Read the model definition and answer for the solid it produces. Units are mm, in the model's axes. A direction names the side the tool comes from. Give positions to 0.01 mm unless a question says otherwise; leave off trailing zeros. Order: outer loops, then holes, each group sorted by start corner. A loop starts at its lowest first (then second) coordinate and runs counter-clockwise, first axis right, second up. Notation, with made-up numbers: (50, 37.5) - (76, 37.5) arc R29 ccw to (76, 65.5) - close; hole circle Ø3 at (-17, 55.5). An arc over 180 degrees is marked (long way). Answer as CSV lines item,"result". Start each with the question number.
from build123d import *

# Parameters (mm, degrees)
F0_R     = 1.5
F1_DEPTH = 3
F3_DEPTH = 6
F4_R     = 1.5
F5_DEPTH = 25
F7_DEPTH = 25


with BuildPart() as f1:
    # F0 (on Front) → F1 (new body)
    with BuildSketch(Plane.XZ):
        Polygon((16.378661, 45), (0, 0), (40, 0), (46.378661, 45), align=None)
        with Locations((19.878661, 41.5)):
            Circle(F0_R, mode=Mode.SUBTRACT)
        with BuildLine():
            ThreePointArc((43.378661, 41.5), (42.577917, 35.417752), (40.230258, 29.75))
            ThreePointArc((40.230258, 29.75), (38.181219, 29.200962), (37.632181, 31.25))
            ThreePointArc((37.632181, 31.25), (39.68014, 36.19421), (40.378661, 41.5))
            ThreePointArc((40.378661, 41.5), (41.878661, 43), (43.378661, 41.5))
        make_face(mode=Mode.SUBTRACT)
    extrude(amount=F1_DEPTH)

    # F2 (on face) → F3 (join)
    with BuildSketch(Plane(origin=(0, 0, 0), x_dir=(-1, 0, 0), z_dir=(0, 1, 0))):
        Polygon((-40.425244, 3), (-40, 0), (-2, 0), (-2, 3), align=None)
    extrude(amount=F3_DEPTH)

    # F4 (on face) → F5 (cut)
    with BuildSketch(Plane(origin=(0, 0, 0), x_dir=(1, 0, 0), z_dir=(0, 0, -1))):
        with Locations((37, -3)):
            Circle(F4_R)
        with Locations((5, -3)):
            Circle(F4_R)
    extrude(amount=-F5_DEPTH, mode=Mode.SUBTRACT)

    # F6 (on face) → F7 (cut)
    with BuildSketch(Plane.XZ.offset(3)):
        Polygon((18.830264, 34.192898), (8.568888, 6), (26.311674, 6), align=None)
        Polygon((40, 21), (22.968705, 34.192898), (30.450115, 6), (35.450115, 6), align=None)
        with BuildLine():
            ThreePointArc((24.878661, 41.5), (24.70829, 40.205905), (24.208788, 39))
            Line((24.208788, 39), (34.601092, 33))
            ThreePointArc((34.601092, 33), (36.2994, 37.100076), (36.878661, 41.5))
            Line((36.878661, 41.5), (24.878661, 41.5))
        make_face()
    extrude(amount=-F7_DEPTH, mode=Mode.SUBTRACT)


with BuildPart() as f8_1:
    # F8: instance of F1
    add(f1.part.mirror(Plane(origin=(24.806781, -3, 21.611158), x_dir=(1, 0, 0), z_dir=(0, -1, 0))))


solid = f8_1.part
(1) Determine the mould class of faces 4 (the flat face through (20, -7, 0)), 5 (the flat face through (8.3, -4.5, 22.8)), 6 (the cylindrical face through (41.85, -4.52, 43)), 7 (the flat face through (21, -12, 2)) for opening direction Z: released by +Z, released by -Z, zero draft, split by the parting line, or undercut.
(2) Section C-C, the plane x = 15 is taken. Write down the section's boundary in (y, z), and give its area (3 significant figures).
(3) Flat-ended cylindrical pins translate along their axes: pin 1 Ø2.5 at (x, y) = (29, -4) entering from -Z; pin 2 Ø2.5 at (x, y) = (5, -9) entering from -Z; pin 3 Ø1.5 at (y, z) = (-4, 15.5) entering from -X; pin 4 Ø8 at (x, z) = (14.5, 17) entering from -Y. Find the tip coordinate at first contact, or state that the pin passes through.
(4) Section D-D, the plane z = 16 is taken. Write down the section's boundary in (x, y).
(5) Straight lines are drawn through the part: line 1 (Y direction, x = 5, z = 1); line 2 (Z direction, x = 33.5, y = -5.25); line 3 (Y direction, x = 16.5, z = 34). For each, find the intervals that lie inside material, in ascending order. Write a range as [from, to].
(6) Section B-B, the plane z = 32 is taken. Write down the section's boundary in (x, y).
(7) Which of the six approach directions +Z, -Z, +X, -X, +Y, -Y give full straight-line access (tool end or side, diameter ignored) to faces 1 (the flat face through (23, -3, 23)), 2 (the cylindrical face through (39.66, -4.52, 36.12)), 3 (the flat face through (21, -9, 3))?
(8) Section A-A, the plane y = -9 is taken. Write down the section's boundary in (x, z).
Checks:
1,face 4,"released by -Z"
1,face 5,"released by +Z"
1,face 6,"undercut"
1,face 7,"zero draft"
2,outline,"(-12, 0) - (-3, 0) - (-3, 6) - (-6, 6) - (-6, 3) - (-12, 3) - close; (-6, 23.67) - (-3, 23.67) - (-3, 41.21) - (-6, 41.21) - close"
2,area,"88.6 mm²"
3,pin 1,"stops at z = 0"
3,pin 2,"passes through"
3,pin 3,"stops at x = 5.37"
3,pin 4,"stops at y = -6"
4,outline,"(5.82, -6) - (12.21, -6) - (12.21, -3) - (5.82, -3) - close; (23.66, -6) - (27.8, -6) - (27.8, -3) - (23.66, -3) - close; (38.48, -6) - (42.27, -6) - (42.27, -3) - (38.48, -3) - close"
5,line 1,"y = [-12, -10.5], [-7.5, -3]"
5,line 2,"z = [0, 6], [26.04, 33.64], [41.5, 45]"
5,line 3,"y = [-6, -3]"
6,outline,"(11.65, -6) - (18.03, -6) - (18.03, -3) - (11.65, -3) - close; (19.41, -6) - (23.55, -6) - (23.55, -3) - (19.41, -3) - close; (25.8, -6) - (38.04, -6) - (38.04, -3) - (25.8, -3) - close; (41.37, -6) - (44.54, -6) - (44.54, -3) - (41.37, -3) - close"
7,face 1,"+Z, -Z, +X, -X, +Y"
7,face 2,"+Y, -Y"
7,face 3,"+Z, +X, -X, -Y"
8,outline,"(2, 0) - (3.5, 0) - (3.5, 3) - (2, 3) - close; (6.5, 0) - (35.5, 0) - (35.5, 3) - (6.5, 3) - close; (38.5, 0) - (40, 0) - (40.43, 3) - (38.5, 3) - close"
